Could you check a few things on this drawing? It's one solid part, dimensions in mm from its lowest x, y, z. A direction names the side the tool comes from. Give positions to 0.01 mm unless a question says otherwise; leave off trailing zeros. Order: outer loops, then holes, each group sorted by start corner. A loop starts at its lowest first (then second) coordinate and runs counter-clockwise, first axis right, second up.
(1) Imagine slicing it at D-D, the plane z = 50.8. Write out the boundary of the cut face in (x, y).
(2) Imagine slicing it at C-C, the plane z = 27. Write out the boundary of the cut face in (x, y).
(3) Imagine slicing it at B-B, the plane y = 83.82. Write out the boundary of the cut face in (x, z), then the cut area to 3 significant figures.
(4) If I drill on probe 1 along Z at (x, y) = (17, 1); probe 2 along Z at (x, y) = (50.8, 99.95); probe 3 along Y at (x, z) = (83.82, 100), over which ranges is the centre line in solid material (lowest first)?
(5) If we mould it in two halves opening along Z, with no side actions, what happens to the marked faces 1, 2 and 3? For each: released by +Z, released by -Z, zero draft, split by the parting line, or undercut.
(6) Will these pins go through, and if not, where does the flat tip stop? pin 1 (7.5 mm diameter, centred on x = 85.5, y = 20, fed in from +Z); pin 2 (15 mm diameter, centred on y = 17.78, z = 83.82, fed in from +X); pin 3 (20.5 mm diameter, centred on x = 83.82, z = 50.8, fed in from -Y).
(7) On a 3-axis mill with a long thin cutter (end or side, diameter ignored), from which of +Z, -Z, +X, -X, +Y, -Y can I reach the whole of each face in a straight line? I mean the marked faces 4, 5, 6, 7 and 8. Say none if no direction works.
(8) Imagine slicing it at A-A, the plane x = 83.82. Write out the boundary of the cut face in (y, z).
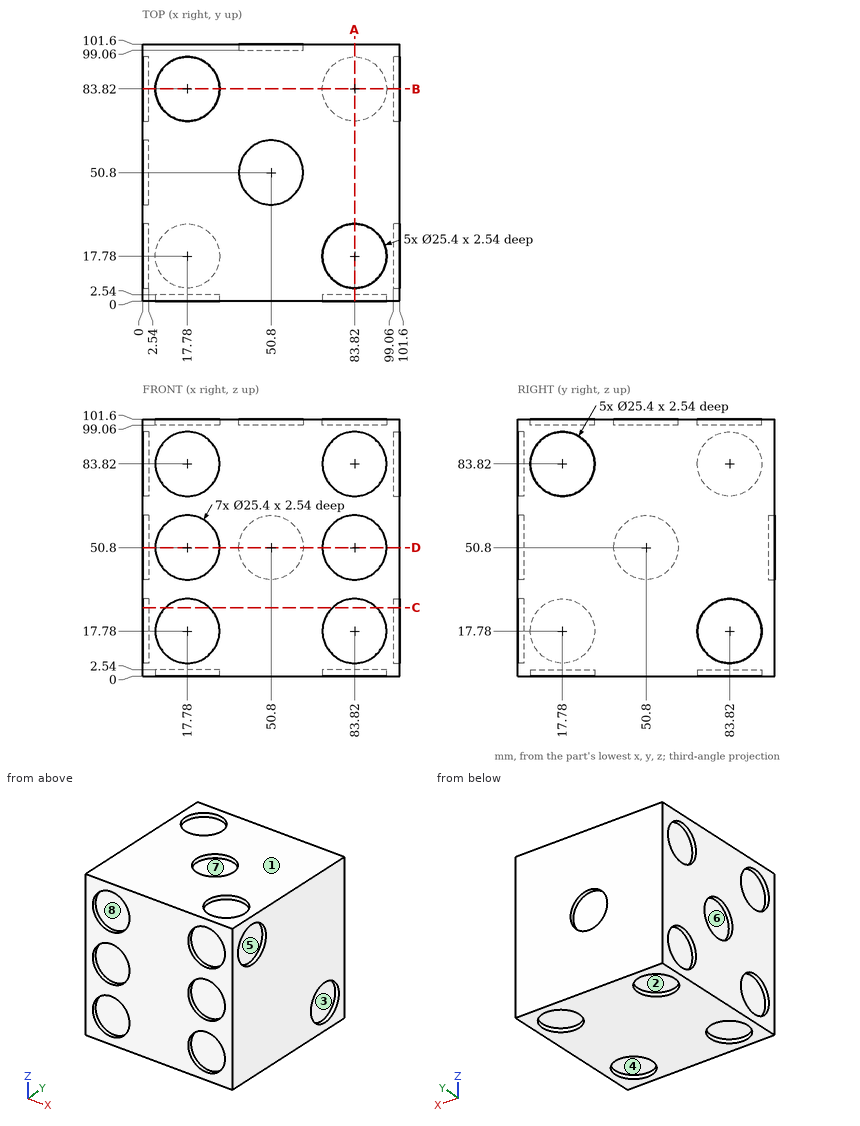
Answer block:
1. outline: (0, 0) - (5.08, 0) - (5.08, 2.54) - (30.48, 2.54) - (30.48, 0) - (71.12, 0) - (71.12, 2.54) - (96.52, 2.54) - (96.52, 0) - (101.6, 0) - (101.6, 101.6) - (63.5, 101.6) - (63.5, 99.06) - (38.1, 99.06) - (38.1, 101.6) - (0, 101.6) - (0, 63.5) - (2.54, 63.5) - (2.54, 38.1) - (0, 38.1) - close
2. outline: (0, 0) - (9.05, 0) - (9.05, 2.54) - (26.51, 2.54) - (26.51, 0) - (75.09, 0) - (75.09, 2.54) - (92.55, 2.54) - (92.55, 0) - (101.6, 0) - (101.6, 75.09) - (99.06, 75.09) - (99.06, 92.55) - (101.6, 92.55) - (101.6, 101.6) - (0, 101.6) - (0, 92.55) - (2.54, 92.55) - (2.54, 75.09) - (0, 75.09) - (0, 26.51) - (2.54, 26.51) - (2.54, 9.05) - (0, 9.05) - close
3. outline: (0, 0) - (5.08, 0) - (5.08, 2.54) - (30.48, 2.54) - (30.48, 0) - (71.12, 0) - (71.12, 2.54) - (96.52, 2.54) - (96.52, 0) - (101.6, 0) - (101.6, 5.08) - (99.06, 5.08) - (99.06, 30.48) - (101.6, 30.48) - (101.6, 101.6) - (30.48, 101.6) - (30.48, 99.06) - (5.08, 99.06) - (5.08, 101.6) - (0, 101.6) - (0, 96.52) - (2.54, 96.52) - (2.54, 71.12) - (0, 71.12) - (0, 30.48) - (2.54, 30.48) - (2.54, 5.08) - (0, 5.08) - close
3. area: 9,940 mm2
4. probe 1: z = 0 to 5.1, 30.46 to 38.12, 63.48 to 71.14, 96.5 to 101.6
4. probe 2: z = 0 to 38.1, 63.5 to 101.6
4. probe 3: y = 0 to 5.08, 30.48 to 101.6
5. face 1: released by +Z
5. face 2: released by -Z
5. face 3: undercut
6. pin 1: stops at z = 99.06
6. pin 2: stops at x = 99.06
6. pin 3: stops at y = 2.54
7. face 4: -Z
7. face 5: +X
7. face 6: -X
7. face 7: +Z
7. face 8: -Y
8. outline: (0, 0) - (5.08, 0) - (5.08, 2.54) - (30.48, 2.54) - (30.48, 0) - (71.12, 0) - (71.12, 2.54) - (96.52, 2.54) - (96.52, 0) - (101.6, 0) - (101.6, 101.6) - (30.48, 101.6) - (30.48, 99.06) - (5.08, 99.06) - (5.08, 101.6) - (0, 101.6) - (0, 96.52) - (2.54, 96.52) - (2.54, 71.12) - (0, 71.12) - (0, 63.5) - (2.54, 63.5) - (2.54, 38.1) - (0, 38.1) - (0, 30.48) - (2.54, 30.48) - (2.54, 5.08) - (0, 5.08) - close
